The drawing under review shows one solid part. Ordinate dimensions are in mm from its lowest x, y, z. Give positions to 0.01 mm unless a question says otherwise; leave off trailing zeros. Order: outer loops, then holes, each group sorted by start corner. A loop starts at its lowest first (then second) coordinate and runs counter-clockwise, first axis right, second up. Notation, with made-up numbers: (-23.75, 8.5) - (-12.75, 8.5) arc R6 ccw to (-12.75, 19.5) - close; hole circle Ø9 at (-28.5, -6). An arc over 180 degrees is marked (long way). Use CSV: the item, a comma, the result in double quotes. Start each with the question number.
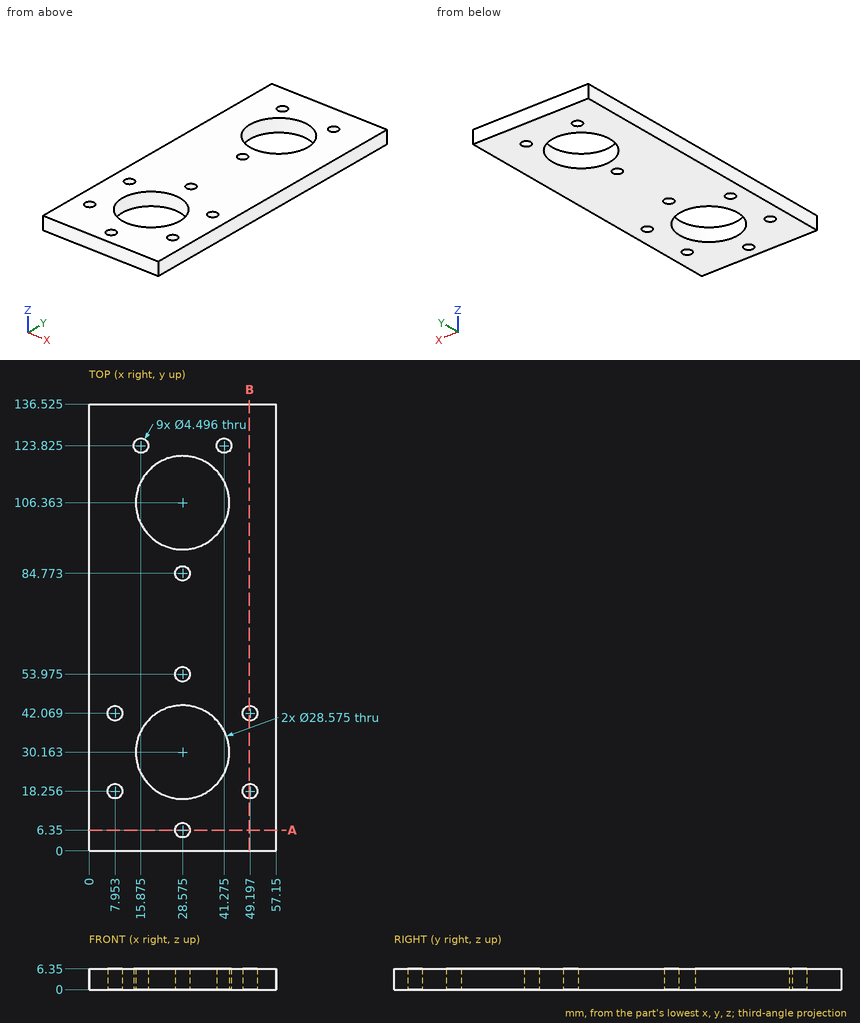
1. To check wall thickness, follow L1, parallel to Y at x = 50.5, z = 4 (1 decimal); L2, parallel to Y at x = 37.5, z = 4.75 (1 decimal); L3, parallel to Y at x = 41, z = 6.25 (1 decimal). State the ranges of each line that lie inside material, in increasing order. Write a range as [from, to].
2. Consider section B-B (x = 49). State how many separate pieces and enclosed holes the cut face has, and give its area (3 significant figures).
3. Consider section A-A (y = 6.35). Give the boundary of the cut face in (x, z), and give its area (3 significant figures).
Answers follow:
1,L1,"y = [0, 16.4], [20.1, 40.2], [43.9, 136.5]"
1,L2,"y = [0, 19], [41.3, 95.2], [117.5, 136.5]"
1,L3,"y = [0, 23.1], [37.2, 99.3], [113.4, 121.6], [126.1, 136.5]"
2,separate pieces,"3"
2,enclosed holes,"0"
2,area,"810 mm^2"
3,outline,"(0, 0) - (26.33, 0) - (26.33, 6.35) - (0, 6.35) - close; (30.82, 0) - (57.15, 0) - (57.15, 6.35) - (30.82, 6.35) - close"
3,area,"334 mm^2"
